Design review of the part built by this model. Coordinates are the model's own, in mm. A direction names the side the tool comes from. Round coordinates to 2 decimals unless told otherwise and drop trailing zeros. Loops run counter-clockwise (first coordinate to the right, second up) from the corner with the lowest first, then second, coordinate; pieces in that order, holes last. Notation, with made-up numbers: (-15, 11) - (18, 11) arc R28 cw to (18, 37) - close; hole circle Ø2 at (31, -10.75). An arc over 180 degrees is marked (long way). Use one line per item in the form item = value. Start each with the question number.
(1) Machinability: for faces 4 (the flat face through (-11, 0, -39.158)), 5 (the flat face through (-10, 0, -43.158)), which of the approach directions +Z, -Z, +X, -X, +Y, -Y give a long, thin tool a straight path to every point of the face, cutting with its end or side? Answer none if there is none.
(2) Wall thickness on probe 1 along Z at (x, y) = (-4, 13.5); probe 2 along X at (y, z) = (14, -36.5); probe 3 along Y at (x, z) = (7.5, -24): over which ranges is each line inside the solid? List them lowest first. Write a range as [from, to].
(3) We need section A-A, the plane y = -15. Write out the cut boundary in (x, z).
(4) The part is to be moulded in two halves that separate along Z. For faces 1 (the flat face through (7.2, 31, -26)), 2 (the cylindrical face through (8.902, 14.425, 13.957)), 3 (the flat face through (8.9, -24.59, 12.25)), say which applies: released by +Z, released by -Z, zero draft, split by the parting line, or undercut.
(5) We need section C-C, the plane y = -3. Write out the cut boundary in (x, z), then the cut area to 3 significant figures.
(6) For pin 1 (3.5 mm diameter, centred on y = -15, z = -22.66, fed in from -X); pin 2 (8 mm diameter, centred on x = -19.5, y = 8, fed in from +Z), all flat-tipped, find the tip position at first contact; note any pin that passes through.
(7) We need section D-D, the plane x = -19. Write out the cut boundary in (y, z).
(8) We need section B-B, the plane z = -23. Write out the cut boundary in (x, y), then the cut area to 3 significant figures.
from build123d import *

# Parameters (mm, degrees)
EXTRUDE_1_DEPTH     = 31
SKETCH_2_R          = 1.5
CUT_EXTRUDE_2_DEPTH = 10


with BuildPart() as part:
    # 草图1 → 凸台-拉伸1 (new, symmetric)
    with BuildSketch(Plane(origin=(0, 0, 0), x_dir=(1, 0, 0), z_dir=(0, 1, 0))):
        Polygon((-30.126027397, 43.157534247), (10.873972603, 43.157534247), (10.873972603, -18.842465753), (6.873972603, -18.842465753), (6.873972603, 39.157534247), (-30.126027397, 39.157534247), align=None)
    extrude(amount=EXTRUDE_1_DEPTH, both=True)

    # 草图2 → 切除-拉伸2 (cut)
    with BuildSketch(Plane(origin=(10.873972603, 0, 0), x_dir=(0, 0, -1), z_dir=(1, 0, 0))):
        Polygon((-5.842465753, 31), (-18.842465753, 31), (-18.842465753, 18), align=None)
        with Locations((22.657534247, -15)):
            Circle(SKETCH_2_R)
        Polygon((-5.842465753, -31), (-18.842465753, -18), (-18.842465753, -31), align=None)
        with Locations((22.657534247, 15)):
            Circle(SKETCH_2_R)
        with Locations((-15.342465753, 15)):
            Circle(SKETCH_2_R)
        with Locations((-15.342465753, -15)):
            Circle(SKETCH_2_R)
    extrude(amount=-CUT_EXTRUDE_2_DEPTH, mode=Mode.SUBTRACT)


solid = part.part
Data:
q1.face_4 = +Z, -X, +Y, -Y
q1.face_5 = -Z, +X, -X, +Y, -Y
q2.probe_1 = [-43.16, -39.16]
q2.probe_2 = [6.87, 10.87]
q2.probe_3 = [-31, -15.67], [-14.33, 14.33], [15.67, 31]
q3.outline = (-30.13, -43.16) - (10.87, -43.16) - (10.87, -24.16) - (6.87, -24.16) - (6.87, -39.16) - (-30.13, -39.16) - close; (6.87, -21.16) - (10.87, -21.16) - (10.87, 13.84) - (6.87, 13.84) - close; (6.87, 16.84) - (10.87, 16.84) - (10.87, 18.84) - (6.87, 18.84) - close
q4.face_1 = zero draft
q4.face_2 = undercut
q4.face_3 = released by +Z
q5.outline = (-30.13, -43.16) - (10.87, -43.16) - (10.87, 18.84) - (6.87, 18.84) - (6.87, -39.16) - (-30.13, -39.16) - close
q5.area = 396 mm^2
q6.pin_1 = 6.87
q6.pin_2 = -39.16
q7.outline = (-31, -43.16) - (31, -43.16) - (31, -39.16) - (-31, -39.16) - close
q8.outline = (6.87, -31) - (10.87, -31) - (10.87, -16.46) - (6.87, -16.46) - close; (6.87, -13.54) - (10.87, -13.54) - (10.87, 13.54) - (6.87, 13.54) - close; (6.87, 16.46) - (10.87, 16.46) - (10.87, 31) - (6.87, 31) - close
q8.area = 225 mm^2
